Verification items for the finished model (mm, model axes). A direction names the side the tool comes from. Give positions to 0.01 mm unless a question says otherwise; leave off trailing zeros. Order: outer loops, then holes, each group sorted by start corner. A loop starts at its lowest first (then second) coordinate and runs counter-clockwise, first axis right, second up. Notation, with made-up numbers: (34, 7) -> (52, 7) arc R19 ccw to (52, 23) -> close; hole circle Ø9 at (-40, -8). An arc over 180 degrees is marked (long way). Return JSON: item names as keys, results as strings. Group by question number.
(1) Depth check by flat-ended pin: pin 1 Ø5.5 at (x, y) = (-10, 0) entering from +Z; pin 2 Ø4.5 at (x, y) = (-27.5, 27.5) entering from +Z; pin 3 Ø1.5 at (x, y) = (21, -10.5) entering from -Z. Enter the tip coordinate at first touch or a pass-through.
(2) Thickness scan on line 1 along X through (y, z) = (-27.5, 0.85); line 2 along Y through (x, z) = (0, 5.7); line 3 along Y through (x, z) = (10, 3). Record the ranges inside material, lowest first.
(3) Cross-section at D-D on y = -10. Enter the section's corners in (x, z).
(4) Tool access check on faces 1 (the face through (22.5, 0, 2)), 2 (the face through (-23.91, -24.02, 6.03)), 3 (the face through (-7, 0, 8)). Record the directions out of +Z, -Z, +X, -X, +Y, -Y that give a thin tool (end or side, any length) a straight path to the whole face; none if there is none.
(5) Cross-section at B-B on z = 2.5. Enter the section's corners in (x, y).
(6) Cross-section at A-A on y = 0. Enter the section's corners in (x, z).
from build123d import *

# Parameters (mm, degrees)
SKETCH1_W           = 63
SKETCH1_H           = 63
BOSS_EXTRUDE1_DEPTH = 8
SKETCH2_W           = 45
SKETCH2_H           = 45
CUT_EXTRUDE1_DEPTH  = 5
SKETCH3_R           = 4.75
CUT_EXTRUDE2_DEPTH  = 5
SKETCH4_R           = 1.75
CUT_EXTRUDE3_DEPTH  = 5
CIRPATTERN1_COUNT   = 4
SKETCH5_R           = 2
CUT_EXTRUDE4_DEPTH  = 15
CIRPATTERN2_COUNT   = 4
FILLET1_R           = 3
SKETCH6_R           = 5
CUT_EXTRUDE5_DEPTH  = 4
CIRPATTERN3_COUNT   = 4
FILLET2_R           = 2
FILLET3_R           = 2


with BuildPart() as part:
    # Sketch1 → Boss-Extrude1 (new body)
    with BuildSketch(Plane.XY):
        Rectangle(SKETCH1_W, SKETCH1_H)
    extrude(amount=BOSS_EXTRUDE1_DEPTH)

    # Sketch2 → Cut-Extrude1 (cut)
    with BuildSketch(Plane(origin=(0, 0, 0), x_dir=(-1, 0, 0), z_dir=(0, 0, -1))):
        Rectangle(SKETCH2_W, SKETCH2_H)
    extrude(amount=-CUT_EXTRUDE1_DEPTH, mode=Mode.SUBTRACT)

    # Sketch3 → Cut-Extrude2 (cut)
    with BuildSketch(Plane.XY.offset(8)):
        Circle(SKETCH3_R)
    extrude(amount=-CUT_EXTRUDE2_DEPTH, mode=Mode.SUBTRACT)

    # Sketch4 → Cut-Extrude3 (cut)
    with BuildSketch(Plane.XY.offset(8)):
        with Locations((0, 10)):
            Circle(SKETCH4_R)
    cut_extrude3 = extrude(amount=-CUT_EXTRUDE3_DEPTH, mode=Mode.SUBTRACT)

    # CirPattern1: Cut-Extrude3 ×4 about axis
    cirpattern1_axis = Axis((0, 0, 0), (0, 0, 1))
    for i in range(1, CIRPATTERN1_COUNT):
        add(cut_extrude3.rotate(cirpattern1_axis, i * 360 / CIRPATTERN1_COUNT), mode=Mode.SUBTRACT)

    # Sketch5 → Cut-Extrude4 (cut)
    with BuildSketch(Plane.XY.offset(8)):
        with Locations((-27.5, 27.5)):
            Circle(SKETCH5_R)
    cut_extrude4 = extrude(amount=-CUT_EXTRUDE4_DEPTH, mode=Mode.SUBTRACT)

    # CirPattern2: Cut-Extrude4 ×4 about axis
    cirpattern2_axis = Axis((0, 0, 0), (0, 0, 1))
    for i in range(1, CIRPATTERN2_COUNT):
        add(cut_extrude4.rotate(cirpattern2_axis, i * 360 / CIRPATTERN2_COUNT), mode=Mode.SUBTRACT)

    # Fillet1
    fillet1_edges = [part.edges().sort_by_distance(p)[0] for p in [
        (-31.5, 31.5, 4),
        (31.5, 31.5, 4),
        (31.5, -31.5, 4),
        (-31.5, -31.5, 4),
    ]]
    fillet(fillet1_edges, radius=FILLET1_R)

    # Sketch6 → Cut-Extrude5 (cut)
    with BuildSketch(Plane.XY.offset(8)):
        with Locations((-27.5, 27.5)):
            Circle(SKETCH6_R)
    cut_extrude5 = extrude(amount=-CUT_EXTRUDE5_DEPTH, mode=Mode.SUBTRACT)

    # CirPattern3: Cut-Extrude5 ×4 about axis
    cirpattern3_axis = Axis((0, 0, 0), (0, 0, 1))
    for i in range(1, CIRPATTERN3_COUNT):
        add(cut_extrude5.rotate(cirpattern3_axis, i * 360 / CIRPATTERN3_COUNT), mode=Mode.SUBTRACT)

    # Fillet2
    fillet2_edges = [part.edges().sort_by_distance(p)[0] for p in [
        (-31.5, 24.5, 6),
        (-24.5, 31.5, 6),
        (31.5, 24.5, 6),
        (24.5, 31.5, 6),
        (24.5, -31.5, 6),
        (31.5, -24.5, 6),
        (-31.5, -24.5, 6),
        (-24.5, -31.5, 6),
    ]]
    fillet(fillet2_edges, radius=FILLET2_R)

    # Fillet3
    fillet3_edges = [part.edges().sort_by_distance(p)[0] for p in [
        (22.5, -22.5, 2.5),
        (22.5, 22.5, 2.5),
        (-22.5, 22.5, 2.5),
        (-22.5, -22.5, 2.5),
    ]]
    fillet(fillet3_edges, radius=FILLET3_R)


solid = part.part
Verdict:
{
 "1": {"pin 1": "z = 8", "pin 2": "z = 4", "pin 3": "z = 5"},
 "2": {"line 1": "-31.5 to -29.5, -25.5 to 25.5, 29.5 to 31.5", "line 2": "-31.5 to -11.75, -8.25 to -4.75, 4.75 to 8.25, 11.75 to 31.5", "line 3": "-31.5 to -22.5, 22.5 to 31.5"},
 "3": {"outline": "(-31.5, 0) -> (-22.5, 0) -> (-22.5, 5) -> (-1.75, 5) -> (-1.75, 8) -> (-31.5, 8) -> close; (1.75, 5) -> (22.5, 5) -> (22.5, 0) -> (31.5, 0) -> (31.5, 8) -> (1.75, 8) -> close"},
 "4": {"face 1": "-Z", "face 2": "+Z", "face 3": "+Z, +X, -X, +Y, -Y"},
 "5": {"outline": "(-31.5, -28.5) arc R3 ccw to (-28.5, -31.5) -> (28.5, -31.5) arc R3 ccw to (31.5, -28.5) -> (31.5, 28.5) arc R3 ccw to (28.5, 31.5) -> (-28.5, 31.5) arc R3 ccw to (-31.5, 28.5) -> close; hole circle Ø4 at (-27.5, -27.5); hole circle Ø4 at (-27.5, 27.5); hole (-22.5, -20.5) arc R2 ccw to (-20.5, -22.5) -> (20.5, -22.5) arc R2 ccw to (22.5, -20.5) -> (22.5, 20.5) arc R2 ccw to (20.5, 22.5) -> (-20.5, 22.5) arc R2 ccw to (-22.5, 20.5) -> close; hole circle Ø4 at (27.5, -27.5); hole circle Ø4 at (27.5, 27.5)"},
 "6": {"outline": "(-31.5, 0) -> (-22.5, 0) -> (-22.5, 5) -> (-11.75, 5) -> (-11.75, 8) -> (-31.5, 8) -> close; (-8.25, 5) -> (-4.75, 5) -> (-4.75, 8) -> (-8.25, 8) -> close; (4.75, 5) -> (8.25, 5) -> (8.25, 8) -> (4.75, 8) -> close; (11.75, 5) -> (22.5, 5) -> (22.5, 0) -> (31.5, 0) -> (31.5, 8) -> (11.75, 8) -> close"}
}
